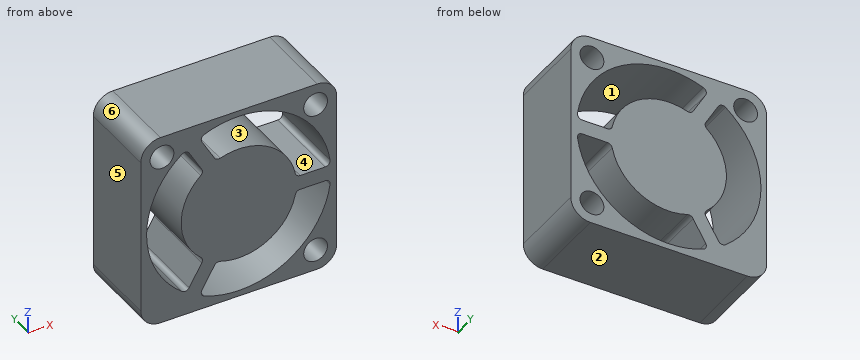
from build123d import *

# Parameters (mm, degrees)
F0_W     = 25.5
F0_H     = 25.5
F1_DEPTH = 10.5
F2_R     = 2.54
F3_R     = 1.55
F4_DEPTH = 10.501


with BuildPart() as f1:
    # F0 (on Front) → F1 (new body)
    with BuildSketch(Plane.XZ):
        Rectangle(F0_W, F0_H)
    extrude(amount=F1_DEPTH)

    # F2
    f2_edges = [f1.edges().sort_by_distance(p)[0] for p in [
        (12.75, -5.25, 12.75),
        (-12.75, -5.25, 12.75),
        (12.75, -5.25, -12.75),
        (-12.75, -5.25, -12.75),
    ]]
    fillet(f2_edges, radius=F2_R)

    # F3 (on face) → F4 (cut, through all)
    with BuildSketch(Plane.XZ.offset(10.5)):
        with Locations((-10, 10)):
            Circle(F3_R)
        with Locations((10, 10)):
            Circle(F3_R)
        with Locations((10, -10)):
            Circle(F3_R)
        with BuildLine():
            ThreePointArc((-4.945405, -5.638526), (-7.5, 0), (-4.945405, 5.638526))
            ThreePointArc((-4.945405, 5.638526), (-4.737594, 6.0125), (-4.81419, 6.433421))
            Line((-4.81419, 6.433421), (-6.451679, 9.269636))
            ThreePointArc((-6.451679, 9.269636), (-6.880602, 9.575501), (-7.392808, 9.452322))
            ThreePointArc((-7.392808, 9.452322), (-12, 0), (-7.392808, -9.452322))
            ThreePointArc((-7.392808, -9.452322), (-6.880602, -9.575501), (-6.451679, -9.269636))
            Line((-6.451679, -9.269636), (-4.81419, -6.433421))
            ThreePointArc((-4.81419, -6.433421), (-4.737594, -6.0125), (-4.945405, -5.638526))
        make_face()
        with BuildLine():
            Line((-4.801901, 10.222136), (-3.164411, 7.385921))
            ThreePointArc((-3.164411, 7.385921), (-2.83818, 7.109127), (-2.410404, 7.102109))
            ThreePointArc((-2.410404, 7.102109), (3.75, 6.495191), (7.355809, 1.463583))
            ThreePointArc((7.355809, 1.463583), (7.575774, 1.096627), (7.978601, 0.9525))
            Line((7.978601, 0.9525), (11.25358, 0.9525))
            ThreePointArc((11.25358, 0.9525), (11.732928, 1.171026), (11.882355, 1.676199))
            ThreePointArc((11.882355, 1.676199), (6, 10.392305), (-4.489547, 11.128521))
            ThreePointArc((-4.489547, 11.128521), (-4.852326, 10.746527), (-4.801901, 10.222136))
        make_face()
        with BuildLine():
            Line((11.25358, -0.9525), (7.978601, -0.9525))
            ThreePointArc((7.978601, -0.9525), (7.575774, -1.096627), (7.355809, -1.463583))
            ThreePointArc((7.355809, -1.463583), (3.75, -6.495191), (-2.410404, -7.102109))
            ThreePointArc((-2.410404, -7.102109), (-2.83818, -7.109127), (-3.164411, -7.385921))
            Line((-3.164411, -7.385921), (-4.801901, -10.222136))
            ThreePointArc((-4.801901, -10.222136), (-4.852326, -10.746527), (-4.489547, -11.128521))
            ThreePointArc((-4.489547, -11.128521), (6, -10.392305), (11.882355, -1.676199))
            ThreePointArc((11.882355, -1.676199), (11.732928, -1.171026), (11.25358, -0.9525))
        make_face()
    extrude(amount=-F4_DEPTH, mode=Mode.SUBTRACT)


solid = f1.part
The listing builds one solid part. Answer for the finished solid, in the listing's coordinates (mm). Face numbers are marked on the shaded views. A direction names the side the tool comes from. Round coordinates to 2 decimals unless told otherwise and drop trailing zeros. Order: outer loops, then holes, each group sorted by start corner. A loop starts at its lowest first (then second) coordinate and runs counter-clockwise, first axis right, second up. Notation, with made-up numbers: (9, 12) -> (59, 12) arc R22 cw to (59, 50) -> close; hole circle Ø3 at (38, -25). An arc over 180 degrees is marked (long way). Put each result on its own line as item: value.
Q1. This flat-tipped pin is pushed along its axis until it touches: P1, Ø2, axis at x = -10, z = -2.5, coming from the -Y side. Where does it stop, or does it pass through?
Results list:
P1: through
Q2. Consider line 1 along Z through (x, y) = (-2.25, -8.75); line 2 along X through (y, z) = (-2.25, -5.75); line 3 along Z through (x, y) = (10.75, -2). Determine where each line is inside the solid, lowest interval first.
Results list:
line 1: -12.75 to -11.79, -7.15 to 7.15, 11.79 to 12.75
line 2: -12.75 to -10.53, -4.85 to 4.82, 10.53 to 12.75
line 3: -12.69 to -11.36, -8.64 to -5.33, -0.95 to 0.95, 5.33 to 8.64, 11.36 to 12.69
Q3. Section C-C, the plane x = -5.5 is taken. Write down the section's boundary in (y, z).
Results list:
outline: (-10.5, -12.75) -> (0, -12.75) -> (0, -7.62) -> (-10.5, -7.62) -> close; (-10.5, -5.1) -> (0, -5.1) -> (0, 5.1) -> (-10.5, 5.1) -> close; (-10.5, 7.62) -> (0, 7.62) -> (0, 12.75) -> (-10.5, 12.75) -> close
Q4. Determine the mould class of the marked faces 3, 4, 5 and 6 for opening direction Z: pulls with the +Z half, pulls with the -Z half, needs draft (parallel to the pull), parting line crosses it, or undercut.
Results list:
face 3: undercut
face 4: undercut
face 5: needs draft
face 6: pulls with the +Z half
Q5. Which of the six approach directions +Z, -Z, +X, -X, +Y, -Y give full straight-line access (tool end or side, diameter ignored) to the marked faces 1 and 2?
Results list:
face 1: +Y, -Y
face 2: -Z, +X, -X, +Y, -Y
Q6. Section A-A, the plane z = 0 is taken. Write down the section's boundary in (x, y), and give its area (4 significant figures).
Results list:
outline: (-12.75, -10.5) -> (-12, -10.5) -> (-12, 0) -> (-12.75, 0) -> close; (-7.5, -10.5) -> (12.75, -10.5) -> (12.75, 0) -> (-7.5, 0) -> close
area: 220.5 mm^2
Q7. Section D-D, the plane x = 1.5 is taken. Write down the section's boundary in (y, z).
Results list:
outline: (-10.5, -12.75) -> (0, -12.75) -> (0, -11.91) -> (-10.5, -11.91) -> close; (-10.5, -7.35) -> (0, -7.35) -> (0, 7.35) -> (-10.5, 7.35) -> close; (-10.5, 11.91) -> (0, 11.91) -> (0, 12.75) -> (-10.5, 12.75) -> close
Q8. Section B-B, the plane x = 9.75 is taken. Write down the section's boundary in (y, z), and give its area (3 significant figures).
Results list:
outline: (-10.5, -12.75) -> (0, -12.75) -> (0, -11.53) -> (-10.5, -11.53) -> close; (-10.5, -8.47) -> (0, -8.47) -> (0, -7) -> (-10.5, -7) -> close; (-10.5, -0.95) -> (0, -0.95) -> (0, 0.95) -> (-10.5, 0.95) -> close; (-10.5, 7) -> (0, 7) -> (0, 8.47) -> (-10.5, 8.47) -> close; (-10.5, 11.53) -> (0, 11.53) -> (0, 12.75) -> (-10.5, 12.75) -> close
area: 76.6 mm^2
